```python
from build123d import *

# Parameters (mm, degrees)
F0_W      = 350.52
F0_H      = 101.6
F1_DEPTH  = 101.6
F3_DEPTH  = 135.89
F4_W      = 56.0828397485
F4_H      = 76.2
F4_W_2    = 126.5943205029
F5_DEPTH  = 86.36
F6_R      = 81.28
F6_W      = 126.5943205029
F6_H      = 12.7
F7_DEPTH  = 214.122
F11_R     = 30.48
F12_R     = 17.78
F13_DEPTH = 25.4


with BuildPart() as f1:
    # F0 (on Top) → F1 (new body)
    with BuildSketch(Plane.XY):
        Rectangle(F0_W, F0_H)
    extrude(amount=F1_DEPTH)

    # F2 (on face) → F3 (cut)
    with BuildSketch(Plane.XZ.offset(50.8)):
        Polygon((-175.26, 101.6), (-175.26, 15.24), (-119.38, 15.24), (-63.2971602515, 101.6), align=None)
        Polygon((175.26, 101.6), (63.2971602515, 101.6), (119.38, 15.24), (175.26, 15.24), align=None)
    extrude(amount=-F3_DEPTH, mode=Mode.SUBTRACT)

    # F4 (on face) → F5 (cut)
    with BuildSketch(Plane.XY.offset(101.6)):
        with Locations((-91.3385801257, 0)):
            Rectangle(F4_W, F4_H)
        Rectangle(F4_W_2, F4_H)
        with Locations((91.3385801257, 0)):
            Rectangle(F4_W, F4_H)
    extrude(amount=-F5_DEPTH, mode=Mode.SUBTRACT)

    # F6 (on face) → F7 (cut)
    with BuildSketch(Plane.XY.offset(101.6)):
        Circle(F6_R)
        with Locations((0, -44.45)):
            Rectangle(F6_W, F6_H, mode=Mode.SUBTRACT)
        with Locations((0, -44.45)):
            Rectangle(F6_W, F6_H)
    extrude(amount=-F7_DEPTH, mode=Mode.SUBTRACT)

    # F8 (on Front) → F10 (revolve)
    with BuildSketch(Plane.XZ):
        Polygon((-81.28, 0), (-20.32, 0), (-20.32, 10.16), (-43.18, 10.16), (-43.18, 15.24), (-68.58, 15.24), (-68.58, 71.12), (-53.34, 71.12), (-53.34, 96.52), (-73.66, 96.52), (-73.66, 101.6), (-81.28, 101.6), align=None)
    revolve(axis=Axis((0, 0, 50.3256209195), (0, 0, 1)))

    # F11
    f11_edges = [f1.edges().sort_by_distance(p)[0] for p in [
        (175.26, -50.8, 7.62),
        (175.26, 50.8, 7.62),
        (-175.26, -50.8, 7.62),
        (-175.26, 50.8, 7.62),
    ]]
    fillet(f11_edges, radius=F11_R)

    # F12 (on face) → F13 (cut)
    with BuildSketch(Plane.XY.offset(15.24)):
        with Locations((-128.27, 0)):
            Circle(F12_R)
        with Locations((128.27, 0)):
            Circle(F12_R)
    extrude(amount=-F13_DEPTH, mode=Mode.SUBTRACT)


solid = f1.part
```
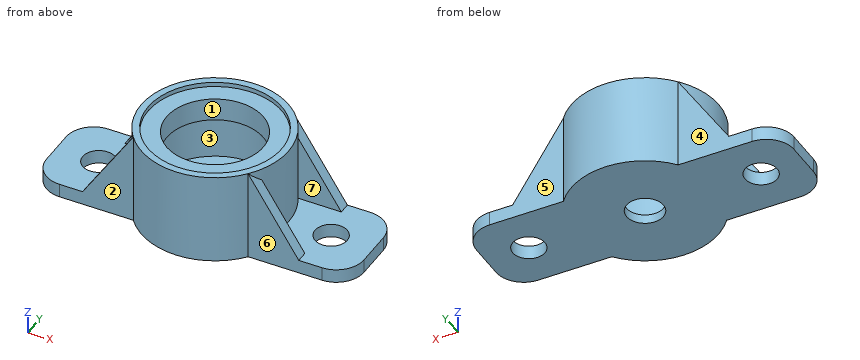
CAD build for the part. Positions are in the model's coordinates, mm. Face numbers are marked on the shaded views. A direction names the side the tool comes from. Give positions to 0.01 mm unless a question says otherwise; leave off trailing zeros. Write each loop counter-clockwise with the first axis right and the second up, starting at its lowest first coordinate (ties: lowest second). Pieces come first, ordered by that corner, then holes. Notation, with made-up numbers: M 14.5,-35.5 L 18.5,-35.5 A21 ccw 18.5,-17.5 Z; hole C 64.5,55.5 d6. An arc over 180 degrees is marked long. Return JSON: item names as keys, results as strings. Group by question number.
(1) Band-saw the part on B-B (z = 47.5). Give the cut face in (x, y).
(2) Band-saw the part on D-D (y = 64). Give the cut face in (x, z), and give its area (3 significant figures).
(3) 3-axis set-ups, long thin cutter, end or side, ignore diameter. For the marked faces 4, 5, 6 and 7: which of +Z, -Z, +X, -X, +Y, -Y reach the whole face in a straight line?
(4) Flat gauge pins, fed straight in: pin 1 Ø1 at (y, z) = (-20.5, 11) entering from -X; pin 2 Ø1 at (x, z) = (-1.5, 54.5) entering from -Y; pin 3 Ø4 at (x, y) = (88.5, 26) entering from +Z; pin 4 Ø8 at (x, z) = (-76, 38) entering from -Y. Where does each tip first touch, or does it go through?
(5) Band-saw the part on C-C (y = 0). State how many separate pieces and enclosed holes the cut face has, and give its area (3 significant figures).
(6) Mould opens along X. For the marked faces 1, 2 and 3 say: pulls with the +X half, pulls with the -X half, needs draft (parallel to the pull), parting line crosses it, or undercut.
(7) Drill centre lines: L1, parallel to X at y = 0, z = 42.5; L2, parallel to Z at x = -36, y = -57.5; L3, parallel to Y at x = 0, z = 99. Where is each one in solid material? Low to high. Write a range as [from, to].
(8) Band-saw the part on A-A (x = 128.27). Give the cut face in (y, z), and give its area (3 significant figures).
Entries:
{
 "1": {"outline": "M -98.43,-50.8 L -63.45,-50.8 A81.28 ccw 63.45,-50.8 L 98.43,-50.8 L 98.43,-38.1 L 71.8,-38.1 A81.28 ccw 71.8,38.1 L 98.43,38.1 L 98.43,50.8 L 63.45,50.8 A81.28 ccw -63.45,50.8 L -98.43,50.8 L -98.43,38.1 L -71.8,38.1 A81.28 ccw -71.8,-38.1 L -98.43,-38.1 Z; hole C 0,0 d137.16"},
 "2": {"outline": "M -50.1,0 L 50.1,0 L 50.1,101.6 L 36.47,101.6 L 36.47,96.52 L -36.47,96.52 L -36.47,101.6 L -50.1,101.6 Z; hole M -24.64,15.24 L 24.64,15.24 L 24.64,71.12 L -24.64,71.12 Z", "area": "7,060 mm^2"},
 "3": {"face 4": "+Z, -Z, -X, +Y", "face 5": "+Z, -Z, +X, +Y", "face 6": "+Z, -Z, +X, -Y", "face 7": "+Z, +X"},
 "4": {"pin 1": "stops at x = -175.26", "pin 2": "stops at y = -81.27", "pin 3": "stops at z = 15.24", "pin 4": "stops at y = -50.8"},
 "5": {"separate pieces": "4", "enclosed holes": "0", "area": "6,320 mm^2"},
 "6": {"face 1": "undercut", "face 2": "needs draft", "face 3": "undercut"},
 "7": {"L1": "x = [-81.28, -68.58], [68.58, 81.28]", "L2": "z = [0, 15.24], [71.12, 96.52]", "L3": "y = [-81.28, -73.66], [73.66, 81.28]"},
 "8": {"outline": "M -50.8,0 L -17.78,0 L -17.78,15.24 L -50.8,15.24 Z; M 17.78,0 L 50.8,0 L 50.8,15.24 L 17.78,15.24 Z", "area": "1,010 mm^2"}
}
